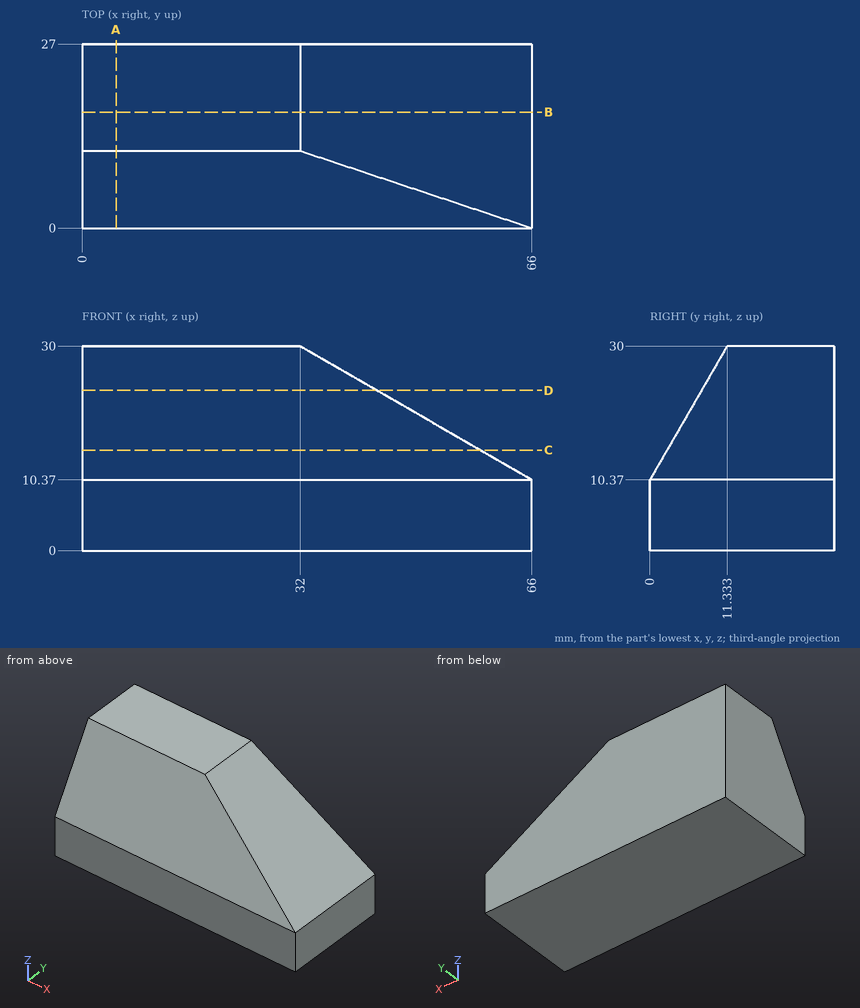
Check sheet for the drawn part. Datum: minimum x, y, z corner. Units: mm. Round coordinates to 2 decimals unless told otherwise and drop trailing zeros. Loops run counter-clockwise (first coordinate to the right, second up) from the corner with the lowest first, then second, coordinate; pieces in that order, holes last.
Item 1: Cross-section at C-C on z = 14.75. Record the boundary of the cut face in (x, y).
Item 2: Cross-section at D-D on z = 23.5. Record the boundary of the cut face in (x, y).
Item 3: Gauge pin test, flat ends, axial feed: pin 1 (8 mm diameter, centred on y = 13, z = 14.5, fed in from +X) (1 decimal); pin 2 (3 mm diameter, centred on x = 28, z = 14.5, fed in from -Y); pin 3 (6 mm diameter, centred on y = 20, z = 22.5, fed in from +X) (1 decimal). Record the tip position at first contact, or that the pin passes through.
Item 4: Thickness scan on line 1 (Z direction, x = 12, y = 9.5) (1 decimal); line 2 (Y direction, x = 30, z = 20.25) (1 decimal); line 3 (Y direction, x = 5, z = 12.5). Record the ranges inside material, lowest first.
Item 5: Cross-section at B-B on y = 17. Record the boundary of the cut face in (x, z).
Item 6: Cross-section at A-A on x = 5. Record the boundary of the cut face in (y, z).
Answer sheet:
1. outline: (0, 2.53) - (58.41, 2.53) - (58.41, 27) - (0, 27) - close
2. outline: (0, 7.58) - (43.26, 7.58) - (43.26, 27) - (0, 27) - close
3. pin 1: stops at x = 65.8
3. pin 2: stops at y = 1.52
3. pin 3: stops at x = 50.2
4. line 1: z = 0 to 26.8
4. line 2: y = 5.7 to 27
4. line 3: y = 1.23 to 27
5. outline: (0, 0) - (66, 0) - (66, 10.37) - (32, 30) - (0, 30) - close
6. outline: (0, 0) - (27, 0) - (27, 30) - (11.33, 30) - (0, 10.37) - close
